```python
from build123d import *

# Parameters (mm, degrees)
SALIENTE_EXTRUIR1_DEPTH    = 19
CROQUIS2_W                 = 9.87256946
CROQUIS2_H                 = 14
CORTAR_EXTRUIR1_DEPTH      = 27
CORTAR_EXTRUIR2_DEPTH      = 11.163106866
CORTAR_EXTRUIR2_DEPTH_BACK = 1.0000001
CROQUIS11_W                = 1
CROQUIS11_H                = 1.020123201
CORTAR_EXTRUIR3_DEPTH      = 33
CROQUIS12_R                = 1.5
SALIENTE_EXTRUIR3_DEPTH    = 3.5
CROQUIS13_W                = 25.1
CROQUIS13_H                = 17
SALIENTE_EXTRUIR5_DEPTH    = 3.5
CROQUIS16_W                = 1
CROQUIS16_H                = 0.5
SALIENTE_EXTRUIR8_DEPTH    = 10.162
CROQUIS19_W                = 1
CROQUIS19_H                = 0.5
SALIENTE_EXTRUIR9_DEPTH    = 10.165


with BuildPart() as part:
    # Croquis1 → Saliente-Extruir1 (new body)
    with BuildSketch(Plane(origin=(0, 0, 0), x_dir=(1, 0, 0), z_dir=(0, 1, 0))):
        with BuildLine():
            Line((0, 30), (0, 0))
            Line((0, 0), (0, -2))
            add(Edge.make_bspline(
                [(0, -2), (0.244064913, -4.453043064), (2.060905279, -6.231862145)],
                knots=[0, 0, 0, 1, 1, 1], degree=2))
            add(Edge.make_bspline(
                [(2.060905279, -6.231862145), (2.507004014, -6.712573557), (2.617207224, -7.344647716)],
                knots=[0, 0, 0, 1, 1, 1], degree=2))
            Line((2.617207224, -7.344647716), (2.617207224, -13.018311654))
            add(Edge.make_bspline(
                [(2.617207224, -13.018311654), (2.630895377, -13.73499915), (3.489917654, -13.737380921)],
                knots=[0, 0, 0, 1, 1, 1], degree=2))
            Line((3.489917654, -13.737380921), (7.744496795, -13.737380921))
            add(Edge.make_bspline(
                [(8.617207224, -13.018311654), (8.603519071, -13.73499915), (7.744496795, -13.737380921)],
                knots=[0, 0, 0, 1, 1, 1], degree=2))
            Line((8.617207224, -13.018311654), (8.617207224, -7.018311654))
            add(Edge.make_bspline(
                [(8.617207224, -7.018311654), (8.52941254, -6.066211773), (9.815332332, -4.707225326), (10.076873528, -2.886889338), (10.163106766, -2)],
                knots=[0, 0, 0, 0, 0.490316762, 1, 1, 1, 1], degree=3))
            Line((10.163106766, -2), (10.163106766, 0))
            Line((10.163106766, 0), (10.163106766, 6.570533479))
            Line((10.163106766, 6.570533479), (3, 30))
            Line((3, 30), (0, 30))
        make_face()
    extrude(amount=SALIENTE_EXTRUIR1_DEPTH)

    # Croquis2 → Cortar-Extruir1 (cut)
    with BuildSketch(Plane(origin=(0, 0, -30), x_dir=(-1, 0, 0), z_dir=(0, 0, -1))):
        with Locations((-7.93628473, 9.5)):
            Rectangle(CROQUIS2_W, CROQUIS2_H)
    extrude(amount=-CORTAR_EXTRUIR1_DEPTH, mode=Mode.SUBTRACT)

    # Croquis10 → Cortar-Extruir2 (cut, two sides)
    with BuildSketch(Plane(origin=(0, 0, 0), x_dir=(0, 0, -1), z_dir=(1, 0, 0))) as cortar_extruir2_sk:
        Polygon((1, 2.5), (1, 16.5), (-13.737380921, 16.5), (-13.737380921, 0), (-1, 0), (-1, 2.5), align=None)
    extrude(amount=CORTAR_EXTRUIR2_DEPTH, mode=Mode.SUBTRACT)
    extrude(cortar_extruir2_sk.sketch, amount=-CORTAR_EXTRUIR2_DEPTH_BACK, mode=Mode.SUBTRACT)

    # Croquis11 → Cortar-Extruir3 (cut)
    with BuildSketch(Plane(origin=(0, 0, 0), x_dir=(0, 0, -1), z_dir=(1, 0, 0))):
        with Locations((0.5, 1.9899384)):
            Rectangle(CROQUIS11_W, CROQUIS11_H)
        with Locations((0.5, 17.010061601)):
            Rectangle(CROQUIS11_W, CROQUIS11_H)
    extrude(amount=CORTAR_EXTRUIR3_DEPTH, mode=Mode.SUBTRACT)

    # Croquis12 → Saliente-Extruir3 (add)
    with BuildSketch(Plane(origin=(0, 19, 0), x_dir=(1, 0, 0), z_dir=(0, 1, 0))):
        with Locations((5.617207224, -10.237380921)):
            Circle(CROQUIS12_R)
    extrude(amount=SALIENTE_EXTRUIR3_DEPTH)

    # Croquis13 → Saliente-Extruir5 (add)
    with BuildSketch(Plane.ZY):
        with Locations((-16.592912937, 9.5)):
            Rectangle(CROQUIS13_W, CROQUIS13_H)
    extrude(amount=SALIENTE_EXTRUIR5_DEPTH)

    # Croquis16 → Saliente-Extruir8 (add)
    with BuildSketch(Plane(origin=(10.163106766, 0, 0), x_dir=(0, 0, -1), z_dir=(1, 0, 0))):
        with Locations((-0.5, 16.25)):
            Rectangle(CROQUIS16_W, CROQUIS16_H)
    extrude(amount=-SALIENTE_EXTRUIR8_DEPTH)

    # Croquis19 → Saliente-Extruir9 (add)
    with BuildSketch(Plane.ZY):
        with Locations((-0.5, 17.270123201)):
            Rectangle(CROQUIS19_W, CROQUIS19_H)
    extrude(amount=-SALIENTE_EXTRUIR9_DEPTH)


solid = part.part
```
Geometry: final body of the model. Coordinates: model frame, mm. A direction names the side the tool comes from. Give positions to 0.01 mm unless a question says otherwise; leave off trailing zeros. Write each loop counter-clockwise with the first axis right and the second up, starting at its lowest first coordinate (ties: lowest second). Pieces come first, ordered by that corner, then holes.
1. Section query C-C, the plane x = -1.5. Return loops of the section in (y, z).
2. Draft query along Z for faces 4 (the flat face through (-2, 18, -17)), 5 (the flat face through (6.63, 1.23, -18.12)), 6 (the flat face through (5, 17.02, -0.5)). Return one class per face: released by +Z, released by -Z, zero draft, split by the parting line, or undercut.
3. Section query A-A, the plane y = 5.5. Return loops of the section in (x, z), then the cut area to 3 significant figures.
4. Pin query (flat end, axial travel): P1, Ø1.2, axis at y = 17, z = 9, coming from the -X side; P2, Ø0.8, axis at x = 7, z = -0.5, coming from the +Y side; P3, Ø4, axis at x = -1.5, y = 8, coming from the +Z side. Return the tip coordinate at first contact, or that it passes through.
5. Reachability of faces 1 (the flat face through (5.2, 16, 0.5)), 2 (the flat face through (-2, 9, -29.143)), 3 (the flat face through (5, 1.48, -0.5)) from +Z, -Z, +X, -X, +Y, -Y: full face, straight path, thin tool, end or side. Return the list, or none.
6. Line query: probe 1 along Y at (x, z) = (3.25, -14); probe 2 along Z at (x, y) = (2.25, 1.75); probe 3 along Y at (x, z) = (3.75, 7). Output: solid intervals per line, ascending.
7. Section query B-B, the plane z = -16.5. Return loops of the section in (x, y).
8. Section query D-D, the plane z = -21. Return loops of the section in (x, y).
Computed:
1. outline: (1, -29.14) - (18, -29.14) - (18, -4.04) - (1, -4.04) - close
2. face 4: zero draft
2. face 5: released by -Z
2. face 6: undercut
3. outline: (-3.5, -29.14) - (0, -29.14) - (0, -30) - (3, -30) - (3, -3) - (10.16, -3) - (10.16, -1) - (0, -1) - (0, -4.04) - (-3.5, -4.04) - close
3. area: 189 mm2
4. P1: stops at x = 2.62
4. P2: stops at y = 19
4. P3: stops at z = -1
5. face 1: +Z, +X, -X
5. face 2: -Z, -X, +Y, -Y
5. face 3: +X, -X
6. probe 1: y = 0 to 2.5, 16.5 to 19
6. probe 2: z = -30 to -1, 0 to 1
6. probe 3: y = 16.5 to 19
7. outline: (-3.5, 1) - (0, 1) - (0, 0) - (7.13, 0) - (7.13, 2.5) - (3, 2.5) - (3, 16.5) - (7.13, 16.5) - (7.13, 19) - (0, 19) - (0, 18) - (-3.5, 18) - close
8. outline: (-3.5, 1) - (0, 1) - (0, 0) - (5.75, 0) - (5.75, 2.5) - (3, 2.5) - (3, 16.5) - (5.75, 16.5) - (5.75, 19) - (0, 19) - (0, 18) - (-3.5, 18) - close
